Design review of the part built by this model. Coordinates are the model's own, in mm. A direction names the side the tool comes from. Coordinates: 2 decimals unless noted, no trailing zeros. Loops run counter-clockwise (first coordinate to the right, second up) from the corner with the lowest first, then second, coordinate; pieces in that order, holes last. Notation, with made-up numbers: (-8.5, 41.5) -> (-2.5, 41.5) arc R21 cw to (-2.5, 57.5) -> close; hole circle Ø4 at (-40, -7.5). An arc over 180 degrees is marked (long way). Answer in a Markdown table with one row per item.
```python
from build123d import *

# Parameters (mm, degrees)
BOSS_EXTRUDE1_DEPTH = 3
SKETCH3_R           = 1
CUT_EXTRUDE1_DEPTH  = 3
SKETCH4_R           = 1
BOSS_EXTRUDE2_DEPTH = 3


with BuildPart() as part:
    # Sketch2 → Boss-Extrude1 (new body)
    with BuildSketch(Plane.XY):
        with BuildLine():
            Line((-17.378860002, -4.822654682), (-13.112961617, -4.822654682))
            ThreePointArc((-13.112961617, -4.822654682), (-11.380910809, -3.822654682), (-9.648860002, -4.822654682))
            Line((-9.648860002, -4.822654682), (-7.642961617, -4.822654682))
            ThreePointArc((-7.642961617, -4.822654682), (-3.910910809, -5.822654682), (-7.642961617, -6.822654682))
            Line((-7.642961617, -6.822654682), (-9.648860002, -6.822654682))
            ThreePointArc((-9.648860002, -6.822654682), (-11.380910809, -7.822654682), (-13.112961617, -6.822654682))
            Line((-13.112961617, -6.822654682), (-17.378860002, -6.822654682))
            ThreePointArc((-17.378860002, -6.822654682), (-21.110910809, -5.822654682), (-17.378860002, -4.822654682))
        make_face()
    extrude(amount=BOSS_EXTRUDE1_DEPTH)

    # Sketch3 → Cut-Extrude1 (cut)
    with BuildSketch(Plane.XY.offset(3)):
        with Locations((-11.380910809, -5.822654682)):
            Circle(SKETCH3_R)
        with Locations((-19.110910809, -5.822654682)):
            Circle(SKETCH3_R)
    extrude(amount=-CUT_EXTRUDE1_DEPTH, mode=Mode.SUBTRACT)

    # Sketch4 → Boss-Extrude2 (add)
    with BuildSketch(Plane(origin=(0, 0, 0), x_dir=(-1, 0, 0), z_dir=(0, 0, -1))):
        with Locations((5.910910809, -5.822654682)):
            Circle(SKETCH4_R)
    extrude(amount=BOSS_EXTRUDE2_DEPTH)


solid = part.part
```
(1) Take a section at D-D on y = -5.6. Give the boundary of the cut face in (x, z).
Evaluation:
| item | result |
|---|---|
| outline | (-21.1, 0) -> (-20.09, 0) -> (-20.09, 3) -> (-21.1, 3) -> close; (-18.14, 0) -> (-12.36, 0) -> (-12.36, 3) -> (-18.14, 3) -> close; (-10.41, 0) -> (-6.89, 0) -> (-6.89, -3) -> (-4.94, -3) -> (-4.94, 0) -> (-3.92, 0) -> (-3.92, 3) -> (-10.41, 3) -> close |
(2) For pin 1 (1.5 mm diameter, centred on x = -13.5, y = -7, fed in from +Z); pin 2 (1.6 mm diameter, centred on x = -9, z = 2, fed in from -Y); pin 3 (1 mm diameter, centred on x = -11.5, y = -5.5, fed in from +Z); pin 4 (3.5 mm diameter, centred on x = -16, z = 1.5, fed in from +Y), all flat-tipped, find the tip position at first contact; note any pin that passes through.
Evaluation:
| item | result |
|---|---|
| pin 1 | stops at z = 3 |
| pin 2 | stops at y = -7.05 |
| pin 3 | passes through |
| pin 4 | stops at y = -4.36 |
(3) Take a section at A-A on y = -6.6. Give the boundary of the cut face in (x, z).
Evaluation:
| item | result |
|---|---|
| outline | (-20.95, 0) -> (-19.74, 0) -> (-19.74, 3) -> (-20.95, 3) -> close; (-18.48, 0) -> (-12.01, 0) -> (-12.01, 3) -> (-18.48, 3) -> close; (-10.75, 0) -> (-6.54, 0) -> (-6.54, -3) -> (-5.28, -3) -> (-5.28, 0) -> (-4.07, 0) -> (-4.07, 3) -> (-10.75, 3) -> close |
(4) Take a section at B-B on z = 0.55. Give the boundary of the cut face in (x, y).
Evaluation:
| item | result |
|---|---|
| outline | (-17.38, -6.82) -> (-13.11, -6.82) arc R2 ccw to (-9.65, -6.82) -> (-7.64, -6.82) arc R2 ccw (long way) to (-7.64, -4.82) -> (-9.65, -4.82) arc R2 ccw to (-13.11, -4.82) -> (-17.38, -4.82) arc R2 ccw (long way) to start; hole circle Ø2 at (-19.11, -5.82); hole circle Ø2 at (-11.38, -5.82) |
(5) To check wall thickness, follow probe 1 along X at (y, z) = (-5.9, 0.25); probe 2 along X at (y, z) = (-4.65, 1.6); probe 3 along Z at (x, y) = (-13.5, -5.2). State the ranges of each line that lie inside material, in increasing order.
Evaluation:
| item | result |
|---|---|
| probe 1 | x = -21.11 to -20.11, -18.11 to -12.38, -10.38 to -3.91 |
| probe 2 | x = -20.73 to -17.49, -13 to -9.76, -7.53 to -4.29 |
| probe 3 | z = 0 to 3 |
(6) Draft analysis for pull direction X (two halves, no side actions). For faces 4 (the cylindrical face through (-6.835, -6.206, -1.479)), 5 (the cylindrical face through (-21.11, -5.9, 1.48)), 6 (the flat face through (-6, -6, -3)), state which applies: pulls with the +X half, pulls with the -X half, needs draft (parallel to the pull), parting line crosses it, or undercut.
Evaluation:
| item | result |
|---|---|
| face 4 | parting line crosses it |
| face 5 | undercut |
| face 6 | needs draft |
(7) Take a section at C-C on x = -9.25. Give the boundary of the cut face in (y, z).
Evaluation:
| item | result |
|---|---|
| outline | (-6.82, 0) -> (-4.82, 0) -> (-4.82, 3) -> (-6.82, 3) -> close |
(8) Tool access review of faces 1 (the flat face through (-15, -4.823, 1)), 2 (the cylindrical face through (-20.11, -5.78, 1.52)), 3 (the flat face through (-9, -6.823, 1)): name each direction out of +Z, -Z, +X, -X, +Y, -Y from which nothing blocks a thin tool from reaching the whole face with its end or side.
Evaluation:
| item | result |
|---|---|
| face 1 | +Z, -Z, +Y |
| face 2 | +Z, -Z |
| face 3 | +Z, -Z, -Y |
